Geometry check sheet. Reference: the model listing, model coordinates, mm. A direction names the side the tool comes from. Coordinates: 2 decimals unless noted, no trailing zeros. Loops run counter-clockwise (first coordinate to the right, second up) from the corner with the lowest first, then second, coordinate; pieces in that order, holes last. Notation, with made-up numbers: (87, 73.5) - (104, 73.5) arc R22 cw to (104, 84.5) - close; hole circle Ø10 at (-5.5, 80). An arc over 180 degrees is marked (long way). Write item = value, one per line. Start each with the question number.
from build123d import *

# Parameters (mm, degrees)
ESQUISSE1_W             = 200
ESQUISSE1_H             = 74
BOSS_EXTRU_1_DEPTH      = 6.35
ESQUISSE3_W             = 6.35
ESQUISSE3_H             = 10.571428572
ENL_V_MAT_EXTRU_1_DEPTH = 6.35
ESQUISSE4_W             = 18.181818182
ESQUISSE4_H             = 6.35
ESQUISSE4_W_2           = 18.181818181
ENL_V_MAT_EXTRU_2_DEPTH = 6.35
ENL_V_MAT_EXTRU_3_DEPTH = 6.35
ENL_V_MAT_EXTRU_4_DEPTH = 6.35


with BuildPart() as part:
    # Esquisse1 → Boss.-Extru.1 (new body)
    with BuildSketch(Plane(origin=(0, 0, 0), x_dir=(1, 0, 0), z_dir=(0, 1, 0))):
        with Locations((0, 37)):
            Rectangle(ESQUISSE1_W, ESQUISSE1_H)
    extrude(amount=BOSS_EXTRU_1_DEPTH)

    # Esquisse3 → Enlèv. mat.-Extru.1 (cut)
    with BuildSketch(Plane(origin=(0, 6.35, 0), x_dir=(1, 0, 0), z_dir=(0, 1, 0))):
        with Locations((-96.825, 15.857142857)):
            Rectangle(ESQUISSE3_W, ESQUISSE3_H)
        with Locations((-96.825, 37)):
            Rectangle(ESQUISSE3_W, ESQUISSE3_H)
        with Locations((-96.825, 58.142857143)):
            Rectangle(ESQUISSE3_W, ESQUISSE3_H)
    enl_v_mat_extru_1 = extrude(amount=-ENL_V_MAT_EXTRU_1_DEPTH, mode=Mode.SUBTRACT)

    # Symétrie1: Enlèv. mat.-Extru.1 across plane
    add(enl_v_mat_extru_1.mirror(Plane(origin=(0, 0, 0), x_dir=(0, 0, 1), z_dir=(1, 0, 0))), mode=Mode.SUBTRACT)

    # Esquisse4 → Enlèv. mat.-Extru.2 (cut)
    with BuildSketch(Plane(origin=(0, 6.35, 0), x_dir=(1, 0, 0), z_dir=(0, 1, 0))):
        with Locations((-90.909090909, 70.825)):
            Rectangle(ESQUISSE4_W, ESQUISSE4_H)
        with Locations((-54.545454546, 70.825)):
            Rectangle(ESQUISSE4_W_2, ESQUISSE4_H)
        with Locations((-18.181818182, 70.825)):
            Rectangle(ESQUISSE4_W, ESQUISSE4_H)
        with Locations((18.181818182, 70.825)):
            Rectangle(ESQUISSE4_W, ESQUISSE4_H)
        with Locations((54.545454546, 70.825)):
            Rectangle(ESQUISSE4_W_2, ESQUISSE4_H)
        with Locations((90.909090909, 70.825)):
            Rectangle(ESQUISSE4_W, ESQUISSE4_H)
    extrude(amount=-ENL_V_MAT_EXTRU_2_DEPTH, mode=Mode.SUBTRACT)

    # Esquisse5 → Enlèv. mat.-Extru.3 (cut)
    with BuildSketch(Plane(origin=(0, 6.35, 0), x_dir=(1, 0, 0), z_dir=(0, 1, 0))):
        with BuildLine():
            Line((-75, 15), (-55, 15))
            ThreePointArc((-55, 15), (-50, 10), (-55, 5))
            Line((-55, 5), (-75, 5))
            ThreePointArc((-75, 5), (-80, 10), (-75, 15))
        make_face()
    enl_v_mat_extru_3 = extrude(amount=-ENL_V_MAT_EXTRU_3_DEPTH, mode=Mode.SUBTRACT)

    # Symétrie2: Enlèv. mat.-Extru.3 across plane
    add(enl_v_mat_extru_3.mirror(Plane(origin=(0, 0, 0), x_dir=(0, 0, 1), z_dir=(1, 0, 0))), mode=Mode.SUBTRACT)

    # Esquisse6 → Enlèv. mat.-Extru.4 (cut)
    with BuildSketch(Plane.XZ):
        with BuildLine():
            Line((-5, 0), (-5, -5))
            ThreePointArc((-5, -5), (0, -10), (5, -5))
            Line((5, -5), (5, 0))
            Line((5, 0), (-5, 0))
        make_face()
    extrude(amount=-ENL_V_MAT_EXTRU_4_DEPTH, mode=Mode.SUBTRACT)


solid = part.part
(1) Depth check by flat-ended pin: pin 1 (1.9 mm diameter, centred on x = 60, y = 1.5, fed in from -Z). Enter the tip coordinate at first touch or a pass-through.
(2) Tool access check on faces 1 (the face through (97, 3, -52.857)), 2 (the face through (-80, 3, -10)), 3 (the face through (91, 3, -67.65)), 4 (the face through (-97, 3, -21.143)). Record the directions out of +Z, -Z, +X, -X, +Y, -Y that give a thin tool (end or side, any length) a straight path to the whole face; none if there is none.
(3) Draft check along X on faces 5 (the face through (45.455, 3, -71)), 6 (the face through (-97, 3, -31.714)), 7 (the face through (93.65, 3, -37)). Enter one of: pulls with the +X half, pulls with the -X half, needs draft (parallel to the pull), parting line crosses it, or undercut.
(4) Scan lines: line 1 (Z direction, x = 63, y = 3.5); line 2 (X direction, y = 3, z = -14); line 3 (X direction, y = 5.25, z = -34). Record each from-to range of solid material in increasing order.
(5) Sectioned sample at C-C on z = -19. Enter the section's corners in (x, y), plus the area to 3 significant figures.
(6) Sectioned sample at A-A on y = 2.75. Count the separate pieces of the cut face and the enclosed holes in it, plus the area to 3 significant figures.
(7) Sectioned sample at B-B on x = 0. Enter the section's corners in (y, z).
Working result:
q1.pin_1 = -67.65
q2.face_1 = +X, +Y, -Y
q2.face_2 = +Y, -Y
q2.face_3 = -Z, +X, +Y, -Y
q2.face_4 = -X, +Y, -Y
q3.face_5 = undercut
q3.face_6 = needs draft
q3.face_7 = pulls with the +X half
q4.line_1 = -67.65 to -15, -5 to 0
q4.line_2 = -93.65 to -78, -52 to 52, 78 to 93.65
q4.line_3 = -93.65 to 93.65
q5.outline = (-93.65, 0) - (93.65, 0) - (93.65, 6.35) - (-93.65, 6.35) - close
q5.area = 1,190 mm2
q6.separate_pieces = 1
q6.enclosed_holes = 2
q6.area = 13,100 mm2
q7.outline = (0, -74) - (6.35, -74) - (6.35, -10) - (0, -10) - close
